Check sheet for the modelled part. Datum: model origin and axes. Units: mm. A direction names the side the tool comes from. Round coordinates to 2 decimals unless told otherwise and drop trailing zeros. Loops run counter-clockwise (first coordinate to the right, second up) from the corner with the lowest first, then second, coordinate; pieces in that order, holes last. Notation, with made-up numbers: (-6, -5.75) -> (17, -5.75) arc R12 cw to (17, 6.25) -> close; hole circle Ø11 at (0, 12.25). An arc over 180 degrees is marked (long way). Use one line per item in the form item = value. Start each with the question number.
(1) Sectioned sample at A-A (x = 20.25). Record the cut outline in (y, z) (3 decimals).
(2) Sectioned sample at B-B (x = 12.5). Record the cut outline in (y, z) (3 decimals).
(3) Go/stop test with a flat-tipped pin: pin 1 (2 mm diameter, centred on x = 16.5, y = -2, fed in from -Z). Record where the tip stops, or that it passes through.
(4) Material ranges on probe 1 along Y at (x, z) = (12.25, -0.1); probe 2 along Y at (x, z) = (19.75, -0.1); probe 3 along Z at (x, y) = (21.5, 2.05), recorded low to high. Write a range as [from, to].
(5) Set-up check for faces 1 (the flat face through (25.286, -0.035, -1.454)), 2 (the cylindrical face through (17.15, 2.32, -0.51)): record each of +Z, -Z, +X, -X, +Y, -Y from which the full face is reachable in a straight line by a thin tool's end or side.
from build123d import *

# Parameters (mm, degrees)
CORTE_EXTRUS_O1_DEPTH = 5
CORTE_EXTRUS_O2_DEPTH = 10
FILETE1_R             = 0.2


with BuildPart() as part:
    # Esboço1 → Revolução1 (revolve)
    with BuildSketch(Plane.XY, mode=Mode.PRIVATE) as revolu_o1_sk:
        Polygon((0, 0), (0, 1.335), (2.836358614, 2.095), (13.09, 2.095), (13.09, 2.375), (21.09, 2.375), (21.09, 2.6), (22.469186813, 2.6), (28.2, 2.6), (28.2, 0), align=None)
    revolve(revolu_o1_sk.sketch.rotate(Axis((0, 0, 0), (1, 0, 0)), 90), axis=Axis((0, 0, 0), (1, 0, 0)))

    # Esboço2 → Corte-extrusão1 (cut, symmetric)
    with BuildSketch(Plane.XY):
        Polygon((28.2, -2.6), (25.943384548, 3.6), (29, 3.6), (29, -2.6), align=None)
    extrude(amount=CORTE_EXTRUS_O1_DEPTH, both=True, mode=Mode.SUBTRACT)

    # Esboço3 → Corte-extrusão2 (cut, along a direction that is not the sketch's normal)
    with BuildSketch(Plane(origin=(-3.863561719, -2.6, 0), x_dir=(0, 0, 1), z_dir=(0, 1, 0))):
        with BuildLine():
            Line((-4.077730135, 25.063561719), (-0.611977577, 31.692934924))
            ThreePointArc((-0.611977577, 31.692934924), (0, 32.063561719), (0.611977577, 31.692934924))
            Line((0.611977577, 31.692934924), (4.077730135, 25.063561719))
            ThreePointArc((4.077730135, 25.063561719), (0, 41.665104992), (-4.077730135, 25.063561719))
        make_face()
    extrude(amount=CORTE_EXTRUS_O2_DEPTH, dir=(-0.3420201433256694, 0.9396926207859082, 0), mode=Mode.SUBTRACT)

    # Filete1
    filete1_edges = [part.edges().sort_by_distance(p)[0] for p in [
        (21.09, 0, -2.6),
    ]]
    fillet(filete1_edges, radius=FILETE1_R)


solid = part.part
Checks:
q1.outline = circle Ø4.75 at (0, 0)
q2.outline = circle Ø4.19 at (0, 0)
q3.pin_1 = -2.15
q4.probe_1 = [-2.09, 2.09]
q4.probe_2 = [-2.37, 2.37]
q4.probe_3 = [-1.6, 1.6]
q5.face_1 = -Z, +X, +Y
q5.face_2 = -X
